Autodesk Inventor part; units mm, degrees
ref_plane "YZ Plane" through (0, 0, 0) normal (1, 0, 0) x (0, 1, 0)
ref_plane "XZ Plane" through (0, 0, 0) normal (0, 1, 0) x (-1, 0, 0)
ref_plane "XY Plane" through (0, 0, 0) normal (0, 0, 1) x (1, 0, 0)
sketch "Sketch1" plane through (0, 0, 0) normal (1, 0, 0) x (0, 1, 0)
  spline S0 degree 3 poles (-21.8, 19) (-21.8911, 18.9704) (-23.5777, 19.1791) (-27.2185, 19.809) (-31.5857, 22.2001) (-34.2433, 25.5665) (-37.0578, 26.9358) (-39.8917, 26.6297) (-42.8949, 26.0623) (-45.8688, 25.4606) (-48.1326, 24.4893) (-48.5091, 23.6382) (-48.5, 23.25) knots 0 0 0 0 0.008681 0.173507 0.363577 0.490264 0.601083 0.655384 0.772555 0.905868 0.967377 1 1 1 1
  line L0 (-48.5, -23.25) -> (-48.5, 23.25)
  arc A0 (-48.5, -23.25) -> (-43.72, -26.1) centre (-43.3877, -20.1092) ccw
  line L1 (-42.92, -26.1) -> (-43.72, -26.1)
  spline S1 degree 3 poles (-36.22, -26.1708) (-32.3391, -21.8472) (-27.5324, -19.457) (-21.8, -19) knots 0 0 0 0 1 1 1 1
  line L2 (-21.8, 19) -> (-21.8, -19)
  line L3 (0, 0) -> (-21.8, 0)
  line L4 (-21.8, 19) -> (-21.8, -19)
  line L5 (-36.22, -26.1708) -> (-37.22, -26.1708)
  line L6 (-37.22, -26.1708) -> (-37.22, -20.4971)
  line L7 (-37.22, -20.4971) -> (-41.92, -20.4971)
  line L8 (-42.92, -26.1) -> (-41.92, -26.1)
  line L9 (-41.92, -26.1) -> (-41.92, -20.4971)
  line L10 (0, 0) -> (0, -18.1714)
  dimension "d0" = 21.8
  dimension "d1" = 38
  dimension "d2" = 1
  dimension "d3" = 1
  dimension "d4" = 4.7
  dimension "d5" = 5.6737
  dimension "d6" = 6
  dimension "d7" = 48.5
revolve "Revolution1" add sketch "Sketch1" angle 360 about axis through (0, 0, 0) along (0, 0, -1)
properties part number "Urethane 97mm" material "Plastic, Opaque Black"
For this review, take the finished solid that the model builds, in its own axes (mm). A direction names the side the tool comes from. Give positions to 0.01 mm unless a question says otherwise; leave off trailing zeros. Write each loop counter-clockwise with the first axis right and the second up, starting at its lowest first coordinate (ties: lowest second). Pieces come first, ordered by that corner, then holes.
Item 1: The part is to be moulded in two halves that separate along Y. For faces 1 (the face through (36, -8, -26.171)), 2 (the face through (-43.028, -22.38, 0.326)), 3 (the face through (-37.5, 0.2, -20.497)), say which applies: +Y half, -Y half, draft (parallel to the pull), parting line (faces both ways), or undercut.
Item 2: Insertion check: P1, Ø1, axis at x = -33.5, y = 15, coming from the +Z side; P2, Ø3, axis at y = -15, z = 12, coming from the -X side; P3, Ø4, axis at x = -1, z = 6, coming from the -Y side; P4, Ø5, axis at x = 17.5, y = -16, coming from the +Z side. Each pin has a flat end and moves straight along its axis. Give the tip position at first contact, or say it passes through.
Item 3: Machinability: for faces 4 (the face through (-6.548, -20.793, -0.266)), 5 (the face through (41.563, 5.457, -23.259)), which of the approach directions +Z, -Z, +X, -X, +Y, -Y give a long, thin tool a straight path to every point of the face, cutting with its end or side? Answer none if there is none.
Item 4: Take a section at A-A (z = 14). Give the boundary of the cut face in (x, y).
Item 5: Wall thickness on probe 1 along Y at (x, z) = (0, -24); probe 2 along Y at (x, z) = (0, -23); probe 3 along X at (y, z) = (0, -22): over which ranges is each line inside the solid? List them lowest first.
Established:
1. face 1: draft
1. face 2: parting line
1. face 3: undercut
2. P1: stops at z = 26.71
2. P2: stops at x = -46.58
2. P3: stops at y = -48.5
2. P4: stops at z = 19.8
3. face 4: +Z, -Z
3. face 5: -Z
4. outline: circle Ø97 at (0, 0); hole circle Ø43.6 at (0, 0)
5. probe 1: y = -47.96 to -41.92, -37.22 to -34.01, 34.01 to 37.22, 41.92 to 47.96
5. probe 2: y = -48.5 to -41.92, -37.22 to -32.75, 32.75 to 37.22, 41.92 to 48.5
5. probe 3: x = -48.5 to -41.92, -37.22 to -31.27, 31.27 to 37.22, 41.92 to 48.5
